Read the model definition and answer for the solid it produces. Units are mm, in the model's axes. Face numbers are marked on the shaded views. Coordinates: 2 decimals unless noted, no trailing zeros. Write each loop counter-clockwise with the first axis right and the second up, starting at its lowest first coordinate (ties: lowest second). Pieces come first, ordered by that corner, then holes. Notation, with made-up numbers: (64, 31.25) - (89, 31.25) arc R9 ccw to (89, 43.25) - close; hole circle Ø6 at (18, 73). An arc over 180 degrees is marked (long way). Use a Markdown table: item, result.
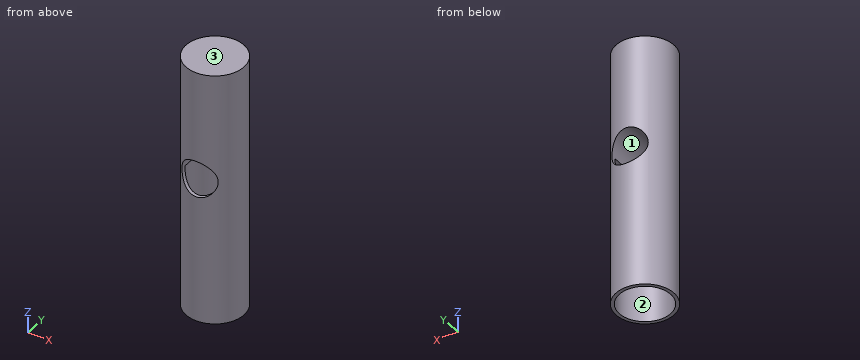
from build123d import *

# Parameters (mm, degrees)
F0_R     = 2.54
F1_DEPTH = 22.225
F5_D     = 3.175
F6_R     = 2.2479
F7_DEPTH = 12.7


with BuildPart() as f1:
    # F0 (on Top) → F1 (new body)
    with BuildSketch(Plane.XY):
        Circle(F0_R)
    extrude(amount=F1_DEPTH)

    # F5 (through all)
    with Locations(Plane.XZ.offset(2.54)):
        with Locations((0, 12.7)):
            Hole(F5_D / 2)

    # F6 (on face) → F7 (cut)
    with BuildSketch(Plane(origin=(0, 0, 0), x_dir=(1, 0, 0), z_dir=(0, 0, -1))):
        Circle(F6_R)
    extrude(amount=-F7_DEPTH, mode=Mode.SUBTRACT)


solid = f1.part
(1) This flat-tipped pin is pushed along its axis until it touches: P1, Ø1, axis at x = 0.5, y = 1, coming from the -Z side. Where does it stop, or does it pass through?
Report:
| item | result |
|---|---|
| P1 | stops at z = 13.93 |
(2) A cutting plane is placed at D-D, the plane z = 19. Write down the section's boundary in (x, y), and give its area (3 significant figures).
Report:
| item | result |
|---|---|
| outline | circle Ø5.08 at (0, 0) |
| area | 20.3 mm² |
(3) A cutting plane is placed at C-C, the plane z = 6. Write down the section's boundary in (x, y), and give its area (3 significant figures).
Report:
| item | result |
|---|---|
| outline | circle Ø5.08 at (0, 0); hole circle Ø4.5 at (0, 0) |
| area | 4.39 mm² |
(4) The mould has two halves that part along Z. Classify the marked faces 1, 2 and 3: pulls with the +Z half, pulls with the -Z half, needs draft (parallel to the pull), parting line crosses it, or undercut.
Report:
| item | result |
|---|---|
| face 1 | undercut |
| face 2 | needs draft |
| face 3 | pulls with the +Z half |
(5) Straight lines are drawn through the part: L1, parallel to Y at x = 0, z = 2.5; L2, parallel to Z at x = 0, y = -0.55 (1 decimal); L3, parallel to Y at x = -1.45, z = 6.5. For each, find the intervals that lie inside material, in ascending order.
Report:
| item | result |
|---|---|
| L1 | y = -2.54 to -2.25, 2.25 to 2.54 |
| L2 | z = 14.3 to 22.2 |
| L3 | y = -2.09 to -1.72, 1.72 to 2.09 |
(6) A cutting plane is placed at A-A, the plane x = 0. Count the separate pieces of the cut face and the enclosed holes in it, and give its area (3 significant figures).
Report:
| item | result |
|---|---|
| separate pieces | 3 |
| enclosed holes | 0 |
| area | 46.8 mm² |
